Part model, mm, in its own coordinate system. Coordinates: 2 decimals unless noted, no trailing zeros. Loops run counter-clockwise (first coordinate to the right, second up) from the corner with the lowest first, then second, coordinate; pieces in that order, holes last. Notation, with made-up numbers: M 78,-32 L 125,-32 A19 ccw 125,-23 Z; hole C 75,-39.75 d5. An arc over 180 degrees is marked long. Answer as a JSON object with one key per item and string values. Group by question number.
1. Drop a flat-ended pin along its axis: pin 1 Ø1 at (x, y) = (47, 1.5) entering from -Z. Give the stop position or say it passes through.
2. Saw through at B-B on x = 12.7. Write the cut outline in (y, z) (3 decimals), then the cut area to 3 significant figures.
3. Saw through at A-A on z = -12.7. Write the cut outline in (x, y) (3 decimals).
4. Drill centre lines: L1, parallel to X at y = 2.3, z = -12.7 (3 decimals); L2, parallel to X at y = 2, z = -38.1; L3, parallel to X at y = 2.5, z = -13.5 (3 decimals). Where is each one in solid material? Low to high.
5. Saw through at C-C on y = 1.3. Write the cut outline in (x, z) (1 decimal), then the cut area to 3 significant figures.
6. Saw through at D-D on z = -24. Write the cut outline in (x, y) (3 decimals), then the cut area to 3 significant figures.
from build123d import *

# Parameters (mm, degrees)
SKETCH1_R           = 2.4892
BOSS_EXTRUDE1_DEPTH = 3.175
FILLET1_R           = 4.7625


with BuildPart() as part:
    # Sketch1 → Boss-Extrude1 (new body)
    with BuildSketch(Plane(origin=(0, 0, 0), x_dir=(1, 0, 0), z_dir=(0, 1, 0))):
        Polygon((0, 0), (0, 60.325), (25.4, 60.325), (25.4, 25.4), (60.325, 25.4), (60.325, 0), align=None)
        with Locations(Location((12.7, 12.7, 0), (0, 0, 270))):
            Circle(SKETCH1_R, mode=Mode.SUBTRACT)
        with Locations(Location((12.7, 25.4, 0), (0, 0, 270))):
            Circle(SKETCH1_R, mode=Mode.SUBTRACT)
        with Locations(Location((12.7, 38.1, 0), (0, 0, 270))):
            Circle(SKETCH1_R, mode=Mode.SUBTRACT)
        with Locations(Location((25.4, 12.7, 0), (0, 0, 270))):
            Circle(SKETCH1_R, mode=Mode.SUBTRACT)
        with Locations(Location((38.1, 12.7, 0), (0, 0, 270))):
            Circle(SKETCH1_R, mode=Mode.SUBTRACT)
        with Locations(Location((50.8, 12.7, 0), (0, 0, 270))):
            Circle(SKETCH1_R, mode=Mode.SUBTRACT)
        with Locations(Location((12.7, 50.8, 0), (0, 0, 270))):
            Circle(SKETCH1_R, mode=Mode.SUBTRACT)
    extrude(amount=BOSS_EXTRUDE1_DEPTH)

    # Fillet1
    fillet1_edges = [part.edges().sort_by_distance(p)[0] for p in [
        (0, 1.5875, 0),
        (0, 1.5875, -60.325),
        (25.4, 1.5875, -60.325),
        (25.4, 1.5875, -25.4),
        (60.325, 1.5875, -25.4),
        (60.325, 1.5875, 0),
    ]]
    fillet(fillet1_edges, radius=FILLET1_R)


solid = part.part
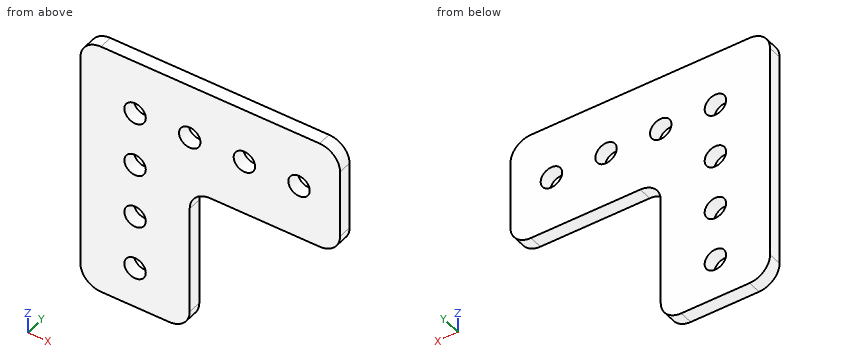
Outcome:
{
 "1": {"pin 1": "stops at z = -25.4"},
 "2": {"outline": "M 0,-60.325 L 3.175,-60.325 L 3.175,-53.289 L 0,-53.289 Z; M 0,-48.311 L 3.175,-48.311 L 3.175,-40.589 L 0,-40.589 Z; M 0,-35.611 L 3.175,-35.611 L 3.175,-27.889 L 0,-27.889 Z; M 0,-22.911 L 3.175,-22.911 L 3.175,-15.189 L 0,-15.189 Z; M 0,-10.211 L 3.175,-10.211 L 3.175,0 L 0,0 Z", "area": "128 mm²"},
 "3": {"outline": "M 0,0 L 10.211,0 L 10.211,3.175 L 0,3.175 Z; M 15.189,0 L 22.911,0 L 22.911,3.175 L 15.189,3.175 Z; M 27.889,0 L 35.611,0 L 35.611,3.175 L 27.889,3.175 Z; M 40.589,0 L 48.311,0 L 48.311,3.175 L 40.589,3.175 Z; M 53.289,0 L 60.325,0 L 60.325,3.175 L 53.289,3.175 Z"},
 "4": {"L1": "x = 0 to 10.211, 15.189 to 22.911, 27.889 to 35.611, 40.589 to 48.311, 53.289 to 60.325", "L2": "x = 0 to 10.21, 15.19 to 25.4", "L3": "x = 0 to 10.343, 15.057 to 23.043, 27.757 to 35.743, 40.457 to 48.443, 53.157 to 60.325"},
 "5": {"outline": "M 0,-55.6 A4.8 ccw 4.8,-60.3 L 20.6,-60.3 A4.8 ccw 25.4,-55.6 L 25.4,-30.2 A4.8 cw 30.2,-25.4 L 55.6,-25.4 A4.8 ccw 60.3,-20.6 L 60.3,-4.8 A4.8 ccw 55.6,0 L 4.8,0 A4.8 ccw 0,-4.8 Z; hole C 12.7,-50.8 d5; hole C 12.7,-38.1 d5; hole C 12.7,-25.4 d5; hole C 12.7,-12.7 d5; hole C 25.4,-12.7 d5; hole C 38.1,-12.7 d5; hole C 50.8,-12.7 d5", "area": "2,260 mm²"},
 "6": {"outline": "M 0,0 L 10.642,0 L 10.642,3.175 L 0,3.175 Z; M 14.758,0 L 58.935,0 L 58.935,3.175 L 14.758,3.175 Z", "area": "174 mm²"}
}
